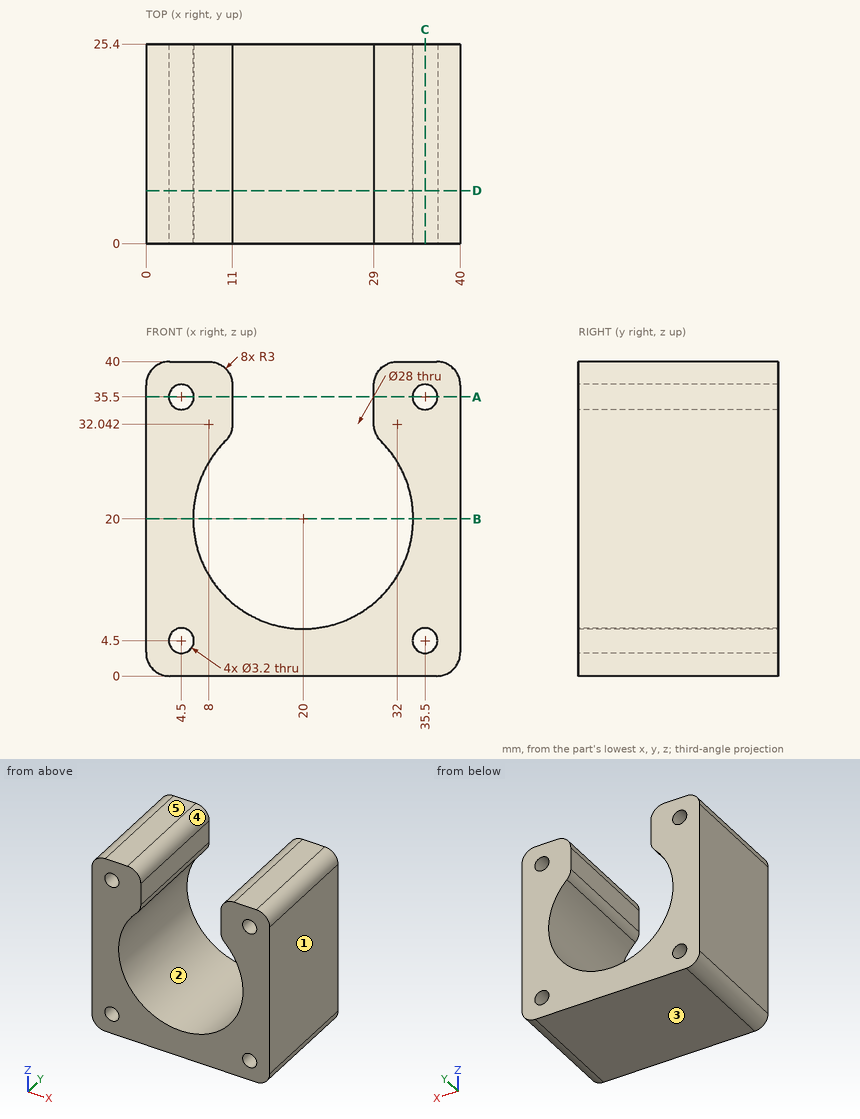
Geometry check sheet. Reference: drawing and pictorial views, mm from the part's lowest x, y, z. A direction names the side the tool comes from. Coordinates: 2 decimals unless noted, no trailing zeros. Order: outer loops, then holes, each group sorted by start corner. A loop starts at its lowest first (then second) coordinate and runs counter-clockwise, first axis right, second up.
Item 1: Tool access check on the marked faces 4 and 5. Record the directions out of +Z, -Z, +X, -X, +Y, -Y that give a thin tool (end or side, any length) a straight path to the whole face; none if there is none.
Item 2: Scan lines: line 1 along X through (y, z) = (20.25, 35.5); line 2 along X through (y, z) = (17.5, 4.5); line 3 along X through (y, z) = (17, 35). Record each from-to range of solid material in increasing order.
Item 3: Section check B-B (z = 20). Enter the section's corners in (x, y), plus the area to 3 significant figures.
Item 4: Section check D-D (y = 6.75). Enter the section's corners in (x, z).
Item 5: Mould release check, pull along Z, two halves, no side actions. Record for the marked faces 1, 2 and 3: released by +Z, released by -Z, zero draft, split by the parting line, or undercut.
Item 6: Section check A-A (z = 35.5). Enter the section's corners in (x, y).
Item 7: Section check C-C (x = 35.5). Enter the section's corners in (y, z).
Check sheet entries:
1. face 4: +Z, +Y, -Y
1. face 5: +Z, +X, -X, +Y, -Y
2. line 1: x = 0 to 2.9, 6.1 to 11, 29 to 33.9, 37.1 to 40
2. line 2: x = 0 to 2.9, 6.1 to 33.9, 37.1 to 40
2. line 3: x = 0 to 2.98, 6.02 to 11, 29 to 33.98, 37.02 to 40
3. outline: (0, 0) - (6, 0) - (6, 25.4) - (0, 25.4) - close; (34, 0) - (40, 0) - (40, 25.4) - (34, 25.4) - close
3. area: 305 mm2
4. outline: (0, 3) arc R3 ccw to (3, 0) - (37, 0) arc R3 ccw to (40, 3) - (40, 37) arc R3 ccw to (37, 40) - (32, 40) arc R3 ccw to (29, 37) - (29, 32.04) arc R3 ccw to (29.88, 29.92) arc R14 cw (long way) to (10.12, 29.92) arc R3 ccw to (11, 32.04) - (11, 37) arc R3 ccw to (8, 40) - (3, 40) arc R3 ccw to (0, 37) - close; hole circle Ø3.2 at (4.5, 4.5); hole circle Ø3.2 at (4.5, 35.5); hole circle Ø3.2 at (35.5, 4.5); hole circle Ø3.2 at (35.5, 35.5)
5. face 1: zero draft
5. face 2: undercut
5. face 3: released by -Z
6. outline: (0, 0) - (2.9, 0) - (2.9, 25.4) - (0, 25.4) - close; (6.1, 0) - (11, 0) - (11, 25.4) - (6.1, 25.4) - close; (29, 0) - (33.9, 0) - (33.9, 25.4) - (29, 25.4) - close; (37.1, 0) - (40, 0) - (40, 25.4) - (37.1, 25.4) - close
7. outline: (0, 0) - (25.4, 0) - (25.4, 2.9) - (0, 2.9) - close; (0, 6.1) - (25.4, 6.1) - (25.4, 33.9) - (0, 33.9) - close; (0, 37.1) - (25.4, 37.1) - (25.4, 40) - (0, 40) - close
